Model file for the job. Use its own axes, mm. A direction names the side the tool comes from. Round coordinates to 2 decimals unless told otherwise and drop trailing zeros. Loops run counter-clockwise (first coordinate to the right, second up) from the corner with the lowest first, then second, coordinate; pieces in that order, holes last. Notation, with made-up numbers: M 35.5,56 L 79.5,56 A26 ccw 79.5,93 Z; hole C 82,88 d8. An arc over 180 degrees is marked long. Answer in a Markdown table with one row per item.
from build123d import *


with BuildPart() as part:
    # Sketch1 → Revolve1 (revolve)
    with BuildSketch(Plane.XY, mode=Mode.PRIVATE) as revolve1_sk:
        with BuildLine():
            Line((0, 1.5875), (0, 26.289))
            Line((0, 26.289), (-1.27, 26.289))
            Line((-1.27, 26.289), (-1.27, 25.3238))
            Line((-1.27, 25.3238), (-9.525, 25.3238))
            Line((-9.525, 25.3238), (-9.525, 17.1958))
            Line((-9.525, 17.1958), (-6.223, 17.1958))
            ThreePointArc((-6.223, 17.1958), (-5.324974388, 16.823825612), (-4.953, 15.9258))
            Line((-4.953, 15.9258), (-4.953, 6.35))
            Line((-4.953, 6.35), (-2.54, 6.35))
            ThreePointArc((-2.54, 6.35), (-1.641974388, 5.978025612), (-1.27, 5.08))
            Line((-1.27, 5.08), (-1.27, 1.5875))
            Line((-1.27, 1.5875), (0, 1.5875))
        make_face()
    revolve(revolve1_sk.sketch.rotate(Axis((0, 0, 0), (-1, 0, 0)), 90), axis=Axis((0, 0, 0), (-1, 0, 0)))  # turned: the seam where the file's is

    # Sketch3 → #8-32 Tapped Hole1 (revolve, cut)
    with BuildSketch(Plane(origin=(-9.525, 20.828, 0), x_dir=(0, 0, 1), z_dir=(0, 1, 0))):
        Polygon((0, 0), (0, 9.525), (2.7178, 9.525), (2.0828, 8.89), (2.0828, 0.635), (2.7178, 0), align=None)
    revolve(axis=Axis((-15.875, 20.828, 0), (1, 0, 0)), mode=Mode.SUBTRACT)


solid = part.part
1. Saw through at C-C (z = 20.5). Write the cut outline in (x, y) (3 decimals), and give its area (3 significant figures).
Verdict:
| item | result |
|---|---|
| outline | M -9.525,-14.868 L -1.27,-14.868 L -1.27,-16.458 L 0,-16.458 L 0,16.458 L -1.27,16.458 L -1.27,14.868 L -9.525,14.868 Z |
| area | 287 mm² |
2. Mould opens along Z. For faces 3 (the flat face through (0, 0, 5)), 4 (the cylindrical face through (-0.644, -7.897, -25.075)), 5 (the cylindrical face through (-3.73, 3.86, 5.04)) say: +Z half, -Z half, draft (parallel to the pull), parting line (faces both ways), or undercut.
Verdict:
| item | result |
|---|---|
| face 3 | draft |
| face 4 | parting line |
| face 5 | undercut |
3. Saw through at D-D (x = -4). Write the cut outline in (y, z), and give its area (3 significant figures).
Verdict:
| item | result |
|---|---|
| outline | C 0,0 d50.65; hole C 0,0 d12.7; hole C 20.83,0 d4.17 |
| area | 1,870 mm² |
4. Pin check, flat tips, straight feed: pin 1 (2 mm diameter, centred on x = -3, y = -6, fed in from -Z); pin 2 (5 mm diameter, centred on x = -1.5, z = -4, fed in from +Y); pin 3 (2 mm diameter, centred on x = -1, z = -10, fed in from -Y). Stop position of each tip, or through.
Verdict:
| item | result |
|---|---|
| pin 1 | stops at z = -24.83 |
| pin 2 | stops at y = 26.25 |
| pin 3 | stops at y = -24.7 |
5. Saw through at A-A (z = 0). State how many separate pieces and enclosed holes the cut face has, and give its area (3 significant figures).
Verdict:
| item | result |
|---|---|
| separate pieces | 3 |
| enclosed holes | 0 |
| area | 238 mm² |
6. Wall check: probe 1 along Y at (x, z) = (-3.4, 0); probe 2 along Y at (x, z) = (-6.5, 0); probe 3 along X at (y, z) = (-18.5, -17.5). Give the ranges that are in metal, low to high.
Verdict:
| item | result |
|---|---|
| probe 1 | y = -25.32 to -6.35, 6.35 to 18.75, 22.91 to 25.32 |
| probe 2 | y = -25.32 to -17.2, 17.2 to 18.75, 22.91 to 25.32 |
| probe 3 | x = -1.27 to 0 |
7. Tool access for faces 1 (the flat face through (-9.525, 5, -17)), 2 (the flat face through (-4.953, 0, -7)): list every direction of +Z, -Z, +X, -X, +Y, -Y with a clear straight run to the whole face (end or side of a thin tool).
Verdict:
| item | result |
|---|---|
| face 1 | +Z, -Z, -X, +Y, -Y |
| face 2 | -X |
